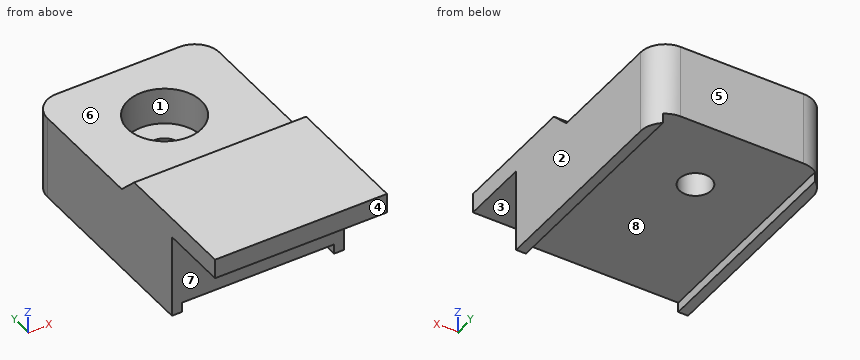
```python
from build123d import *

# Parameters (mm, degrees)
F0_W      = 35
F0_H      = 45
F1_DEPTH  = 15
F2_W      = 2
F2_H      = 45
F3_DEPTH  = 2
F4_W      = 35
F4_H      = 13.8643281162
F4_H_2    = 16.1356718838
F5_DEPTH  = 4
F6_SIZE   = 3.99999
F7_R      = 3.25
F8_DEPTH  = 15
F9_R      = 5
F10_R     = 7.5
F10_R_2   = 3.25
F11_DEPTH = 7.5


# Not quite as in the source:
# - a fillet or chamfer is up to 0.001 mm smaller than in the source, because OpenCascade refuses the exact size


with BuildPart() as f1:
    # F0 (on Top) → F1 (new body)
    with BuildSketch(Plane.XY):
        Rectangle(F0_W, F0_H)
    extrude(amount=F1_DEPTH)

    # F2 (on face) → F3 (join)
    with BuildSketch(Plane(origin=(0, 0, 0), x_dir=(1, 0, 0), z_dir=(0, 0, -1))):
        with Locations((-16.5, 0)):
            Rectangle(F2_W, F2_H)
        with Locations((16.5, 0)):
            Rectangle(F2_W, F2_H)
    extrude(amount=F3_DEPTH)

    # F4 (on face) → F5 (join)
    with BuildSketch(Plane.XY.offset(15)):
        with Locations((0, -29.4321640581)):
            Rectangle(F4_W, F4_H)
        with Locations((0, -14.4321640581)):
            Rectangle(F4_W, F4_H_2)
    extrude(amount=F5_DEPTH)

    # F6 (size 4 in the source; OpenCascade refuses exactly that, so slightly less here)
    f6_edges = [f1.edges().sort_by_distance(p)[0] for p in [
        (0, -6.364328, 19),
    ]]
    chamfer(f6_edges, length=F6_SIZE)

    # F7 (on face) → F8 (cut, through all)
    with BuildSketch(Plane.XY.offset(15)):
        with Locations((0, 7.5)):
            Circle(F7_R)
    extrude(amount=-F8_DEPTH, mode=Mode.SUBTRACT)

    # F9
    f9_edges = [f1.edges().sort_by_distance(p)[0] for p in [
        (-17.5, 22.5, 6.5),
        (17.5, 22.5, 6.5),
    ]]
    fillet(f9_edges, radius=F9_R)

    # F10 (on face) → F11 (cut)
    with BuildSketch(Plane.XY.offset(15)):
        with Locations((0, 7.5)):
            Circle(F10_R)
        with Locations((0, 7.5)):
            Circle(F10_R_2, mode=Mode.SUBTRACT)
    extrude(amount=-F11_DEPTH, mode=Mode.SUBTRACT)


solid = f1.part
```
The listing builds one solid part. Answer for the finished solid, in the listing's coordinates (mm). Face numbers are marked on the shaded views. A direction names the side the tool comes from. Give positions to 0.01 mm unless a question says otherwise; leave off trailing zeros. Loops run counter-clockwise (first coordinate to the right, second up) from the corner with the lowest first, then second, coordinate; pieces in that order, holes last. Notation, with made-up numbers: (13, -3.5) - (51, -3.5) arc R11 cw to (51, 5.5) - close; hole circle Ø6 at (-9.75, 6.25). An arc over 180 degrees is marked (long way). Return JSON: item names as keys, results as strings. Group by question number.
1. Find section B-B (z = 13.5). Write down the section's boundary in (x, y).
2. Find section C-C (y = 7.5). Write down the section's boundary in (x, z), then the cut area to 3 significant figures.
3. Straight lines are drawn through the part: line 1 (Y direction, x = 0, z = 10); line 2 (Y direction, x = 0, z = 4.25); line 3 (Z direction, x = 9, y = -16). For each, find the intervals that lie inside material, in ascending order. Write a range as [from, to].
4. Given pin 1 Ø13.5 at (x, y) = (0, 7.5) entering from +Z; pin 2 Ø4 at (x, y) = (0, 7.5) entering from -Z; pin 3 Ø1.5 at (x, y) = (-4, -28) entering from -Z; pin 4 Ø5 at (x, y) = (6.5, -5) entering from -Z, each flat-ended and moving along its own axis, determine where each tip first touches the part or whether it passes through.
5. Which of the six approach directions +Z, -Z, +X, -X, +Y, -Y give full straight-line access (tool end or side, diameter ignored) to the marked faces 4, 5, 6, 7 and 8?
6. Determine the mould class of the marked faces 1, 2 and 3 for opening direction X: pulls with the +X half, pulls with the -X half, needs draft (parallel to the pull), parting line crosses it, or undercut.
Verdict:
{
 "1": {"outline": "(-17.5, -22.5) - (17.5, -22.5) - (17.5, 17.5) arc R5 ccw to (12.5, 22.5) - (-12.5, 22.5) arc R5 ccw to (-17.5, 17.5) - close; hole circle Ø15 at (0, 7.5)"},
 "2": {"outline": "(-17.5, -2) - (-15.5, -2) - (-15.5, 0) - (-3.25, 0) - (-3.25, 7.5) - (-7.5, 7.5) - (-7.5, 15) - (-17.5, 15) - close; (3.25, 0) - (15.5, 0) - (15.5, -2) - (17.5, -2) - (17.5, 15) - (7.5, 15) - (7.5, 7.5) - (3.25, 7.5) - close", "area": "372 mm^2"},
 "3": {"line 1": "y = [-22.5, 0], [15, 22.5]", "line 2": "y = [-22.5, 4.25], [10.75, 22.5]", "line 3": "z = [0, 19]"},
 "4": {"pin 1": "stops at z = 7.5", "pin 2": "passes through", "pin 3": "stops at z = 15", "pin 4": "stops at z = 0"},
 "5": {"face 4": "+Z, -Z, +X, -X, -Y", "face 5": "+Z, -Z, +X, -X, +Y", "face 6": "+Z, +X, -X, +Y", "face 7": "-Z, +X, -X, -Y", "face 8": "-Z, +Y, -Y"},
 "6": {"face 1": "undercut", "face 2": "pulls with the +X half", "face 3": "needs draft"}
}
